Geometry: final body of the model. Coordinates: model frame, mm. Coordinates: 2 decimals unless noted, no trailing zeros. Write each loop counter-clockwise with the first axis right and the second up, starting at its lowest first coordinate (ties: lowest second). Pieces come first, ordered by that corner, then holes. Notation, with made-up numbers: (74, -27) - (114, -27) arc R16 ccw to (114, -7) - close; hole circle Ø4 at (-19.75, 81.5). An arc over 180 degrees is marked (long way). Answer as a JSON object with one key per item and string values. Group by question number.
Item 1: First-contact query: pin 1 Ø5 at (y, z) = (21.5, 2.5) entering from -X; pin 2 Ø8 at (x, z) = (15, 3.5) entering from +Y; pin 3 Ø2 at (x, z) = (16.5, 9.5) entering from +Y. Flat tips, straight axial feed; report the tip coordinate or a pass-through.
Item 2: Section B-B on x = 16.5. Return loops of the section in (y, z).
Item 3: Section A-A on x = 6.5. Return loops of the section in (y, z).
Item 4: Line query: line 1 along X through (y, z) = (10.75, 6.25); line 2 along X through (y, z) = (13, 6); line 3 along X through (y, z) = (19.5, 5.25). Output: solid intervals per line, ascending. Write a range as from..to.
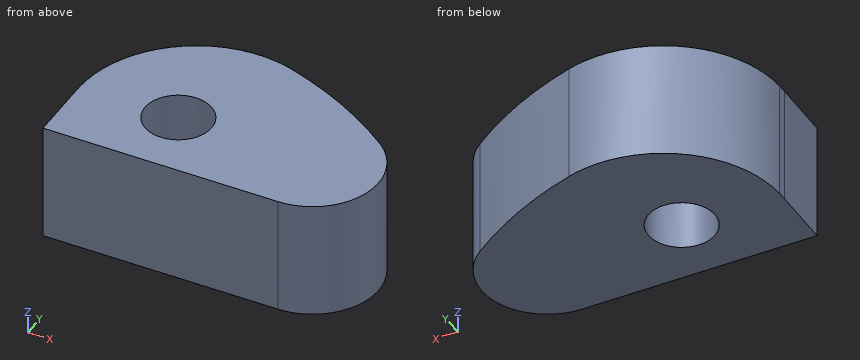
```python
from build123d import *

# Parameters (mm, degrees)
F0_R        = 5.05
F1_DEPTH    = 18
F2_R        = 10
F3_T1_DEPTH = 139.38722981
F4_R        = 9.99999
F5_T1_DEPTH = 121.084516093
F6_R        = 18


# Not quite as in the source:
# - a fillet or chamfer that OpenCascade refuses, or shapes differently, is made with other operations: its cross-section is extruded or revolved along the edge and cut away or added
# - a fillet or chamfer is up to 0.001 mm smaller than in the source, because OpenCascade refuses the exact size


with BuildPart() as f1:
    # F0 (on Top) → F1 (new body)
    with BuildSketch(Plane.XY):
        Polygon((-17.3258748727, 30), (-17.3258748727, 0), (42.6741251273, 0), (12.6741251273, 30), align=None)
        with Locations((-2.3258748727, 10.59)):
            Circle(F0_R, mode=Mode.SUBTRACT)
    extrude(amount=F1_DEPTH)

    # F2
    f2_edges = [f1.edges().sort_by_distance(p)[0] for p in [
        (42.674125, 0, 9),
    ]]
    fillet(f2_edges, radius=F2_R)

    # F3: fillet of radius 60 on 1 edges, made by hand

    # F3_s2 → F3_t1 (cut)
    with BuildSketch(Plane.XY.offset(-60.693614905)):
        with BuildLine():
            ThreePointArc((25.6030573154, 17.0710678119), (8.0910429692, 26.6756740971), (-11.6033208347, 30))
            Line((-11.6033208347, 30), (-11.6033208347, 31.2))
            Line((-11.6033208347, 31.2), (12.6741251273, 31.2))
            Line((12.6741251273, 31.2), (13.5226532647, 30.8485281374))
            ThreePointArc((13.5226532647, 30.8485281374), (19.9871193587, 24.3840620434), (26.3471848784, 18.0124891681))
            Line((26.3471848784, 18.0124891681), (25.6030573154, 17.0710678119))
        make_face()
    extrude(amount=F3_T1_DEPTH, mode=Mode.SUBTRACT)

    # F4 (radius 10 in the source; OpenCascade refuses exactly that, so slightly less here)
    f4_edges = [f1.edges().sort_by_distance(p)[0] for p in [
        (25.603057, 17.071068, 9),
    ]]
    fillet(f4_edges, radius=F4_R)

    # F5: fillet of radius 40 on 1 edges, made by hand

    # F5_s2 → F5_t1 (cut)
    with BuildSketch(Plane.XY.offset(-51.5422580465)):
        with BuildLine():
            ThreePointArc((-17.3258748727, 9.3830967814), (-15.8686941682, 20.0812779708), (-11.6033208347, 30))
            Line((-11.6033208347, 30), (-17.3258748727, 30))
            Line((-17.3258748727, 30), (-17.3258748727, 9.3830967814))
        make_face()
    extrude(amount=F5_T1_DEPTH, mode=Mode.SUBTRACT)

    # F6
    f6_edges = [f1.edges().sort_by_distance(p)[0] for p in [
        (-11.603321, 30, 9),
    ]]
    fillet(f6_edges, radius=F6_R)


solid = f1.part
```
Checks:
{
 "1": {"pin 1": "x = -14.99", "pin 2": "y = 25.58", "pin 3": "y = 23.53"},
 "2": {"outline": "(0, 0) - (23.01, 0) - (23.01, 18) - (0, 18) - close"},
 "3": {"outline": "(0, 0) - (27.2, 0) - (27.2, 18) - (0, 18) - close"},
 "4": {"line 1": "-17.3..-7.37, 2.72..28.37", "line 2": "-17.09..-6.76, 2.11..27.94", "line 3": "-14.7..22.3"}
}
